Read the model definition and answer for the solid it produces. Units are mm, in the model's axes. A direction names the side the tool comes from. Coordinates: 2 decimals unless noted, no trailing zeros. Loops run counter-clockwise (first coordinate to the right, second up) from the corner with the lowest first, then second, coordinate; pieces in that order, holes last.
Q1. A flat-ended cylindrical pin translates along its axis: P1, Ø6, axis at x = -3.5, z = -0.5, coming from the -Y side. Find the tip coordinate at first contact, or state that the pin passes through.
Q2. Which of the six approach directions +Z, -Z, +X, -X, +Y, -Y give full straight-line access (tool end or side, diameter ignored) to faces 4 (the face through (4, -7, 0)), 5 (the face through (-0.96, -21.58, -1.05)), 6 (the face through (-3, -17, 4))?
Q3. Section C-C (x = -3.5) is taken. Give the vertices of the cut face in (y, z).
Q4. The mould has two halves that part along X. Classify faces 1 (the face through (-4, -15, 7.5)), 2 (the face through (-4, -2, 0)), 3 (the face through (-11, -25, 0)): pulls with the +X half, pulls with the -X half, needs draft (parallel to the pull), parting line crosses it, or undercut.
Q5. Straight lines are drawn through the part: line 1 (Y direction, x = -9.5, z = 0.75); line 2 (Z direction, x = -3.5, y = -25.9); line 3 (Y direction, x = -2.25, z = -2.5). For each, find the intervals that lie inside material, in ascending order.
Q6. Section A-A (z = 0) is taken. Give the vertices of the cut face in (x, y).
Q7. Section D-D (z = -6.5) is taken. Give the vertices of the cut face in (x, y).
Q8. Section B-B (y = -23.5) is taken. Give the vertices of the cut face in (x, z), then the cut area to 3 significant figures.
from build123d import *

# Parameters (mm, degrees)
SKETCH1_W           = 15
SKETCH1_H           = 30
BOSS_EXTRUDE1_DEPTH = 7.5
SKETCH2_R           = 5.25
CUT_EXTRUDE1_DEPTH  = 6
SKETCH4_R           = 2.75
CUT_EXTRUDE3_DEPTH  = 28
CUT_EXTRUDE4_REACH  = 36.369
SKETCH5_W           = 8
SKETCH5_H           = 5.1
CHAMFER3_SIZE       = 4


with BuildPart() as part:
    # Sketch1 → Boss-Extrude1 (new, symmetric)
    with BuildSketch(Plane.XY):
        with Locations((-3.5, -15)):
            Rectangle(SKETCH1_W, SKETCH1_H)
    extrude(amount=BOSS_EXTRUDE1_DEPTH, both=True)

    # Sketch2 → Cut-Extrude1 (cut)
    with BuildSketch(Plane.XZ.offset(30)):
        with Locations((-3.5, 0)):
            Circle(SKETCH2_R)
    extrude(amount=-CUT_EXTRUDE1_DEPTH, mode=Mode.SUBTRACT)

    # Sketch4 → Cut-Extrude3 (cut)
    with BuildSketch(Plane.XZ.offset(30)):
        with Locations((-3.5, 0)):
            Circle(SKETCH4_R)
    extrude(amount=-CUT_EXTRUDE3_DEPTH, mode=Mode.SUBTRACT)

    # Sketch5 → Cut-Extrude4 (cut, up to next)
    with BuildSketch(Plane(origin=(4, 0, 0), x_dir=(0, 0, -1), z_dir=(1, 0, 0)), mode=Mode.PRIVATE) as cut_extrude4_sk1:
        with Locations((0, -16.55)):
            Rectangle(SKETCH5_W, SKETCH5_H)
    cut_extrude4_tool1 = extrude(cut_extrude4_sk1.sketch, amount=-CUT_EXTRUDE4_REACH, mode=Mode.PRIVATE) & part.part
    add(cut_extrude4_tool1.solids().sort_by_distance((4, -16.55, 0))[0], mode=Mode.SUBTRACT)

    # Chamfer3
    # the kernel refuses this chamfer: 4 mm, written as the material it takes off along each edge
    with BuildSketch(Plane(origin=(-11, -40.286731952, 7.5), x_dir=(0.9996219169112968, 0, 0.027495876610586275), z_dir=(0, 1, 0)), Plane(origin=(4, 10.286731952, -7.5), x_dir=(0.02749587661058638, 0, 0.9996219169112968), z_dir=(0, -1, 0))) as chamfer3_piece_1:
        Polygon((CHAMFER3_SIZE * 0.999621916911, CHAMFER3_SIZE * 0.0274958766106), (-CHAMFER3_SIZE * 0.0274958766106, CHAMFER3_SIZE * 0.999621916911), (0, 0), align=None)
    extrude(amount=50.573463904, mode=Mode.SUBTRACT)
    with BuildSketch(Plane(origin=(-11, -40.286731952, -7.5), x_dir=(0.9996219169112968, 0, -0.027495876610586275), z_dir=(0, 1, 0)), Plane(origin=(4, 10.286731952, 7.5), x_dir=(0.02749587661058638, 0, -0.9996219169112968), z_dir=(0, -1, 0))) as chamfer3_piece_2:
        Polygon((CHAMFER3_SIZE * 0.999621916911, -CHAMFER3_SIZE * 0.0274958766106), (-CHAMFER3_SIZE * 0.0274958766106, -CHAMFER3_SIZE * 0.999621916911), (0, 0), align=None)
    extrude(amount=50.573463904, mode=Mode.SUBTRACT)


solid = part.part
Numbers:
1. P1: stops at y = -24
2. face 4: +Z, -Z, +X, +Y, -Y
2. face 5: -Y
2. face 6: +X, -X
3. outline: (-30, -7.5) - (0, -7.5) - (0, 7.5) - (-30, 7.5) - (-30, 5.25) - (-24, 5.25) - (-24, 2.75) - (-19.1, 2.75) - (-19.1, 4) - (-14, 4) - (-14, 2.75) - (-2, 2.75) - (-2, -2.75) - (-14, -2.75) - (-14, -4) - (-19.1, -4) - (-19.1, -2.75) - (-24, -2.75) - (-24, -5.25) - (-30, -5.25) - close
4. face 1: needs draft
4. face 2: undercut
4. face 3: pulls with the -X half
5. line 1: y = -30 to -19.1, -14 to 0
5. line 2: z = -7.5 to -5.25, 5.25 to 7.5
5. line 3: y = -24 to -19.1, -14 to 0
6. outline: (-11, -30) - (-8.75, -30) - (-8.75, -24) - (-6.25, -24) - (-6.25, -19.1) - (-11, -19.1) - close; (-11, -14) - (-6.25, -14) - (-6.25, -2) - (-0.75, -2) - (-0.75, -14) - (4, -14) - (4, 0) - (-11, 0) - close; (-0.75, -24) - (1.75, -24) - (1.75, -30) - (4, -30) - (4, -19.1) - (-0.75, -19.1) - close
7. outline: (-8, -30) - (1, -30) - (1, 0) - (-8, 0) - close
8. outline: (-11, -3.5) - (-7, -7.5) - (0, -7.5) - (4, -3.5) - (4, 3.5) - (0, 7.5) - (-7, 7.5) - (-11, 3.5) - close; hole circle Ø5.5 at (-3.5, 0)
8. area: 169 mm2
